from build123d import *

# Parameters (mm, degrees)
SKETCH1_W           = 14.7
SKETCH1_H           = 29.42
SKETCH1_R           = 1.5
SKETCH1_W_2         = 23
SKETCH1_H_2         = 35.5
BOSS_EXTRUDE5_DEPTH = 1.8
SKETCH2_W           = 23
SKETCH2_H           = 35.5
BOSS_EXTRUDE7_DEPTH = 2.6
SKETCH3_R           = 0.510447256
SKETCH3_R_2         = 0.580916902
SKETCH3_R_3         = 0.525090018
CUT_EXTRUDE1_DEPTH  = 1
SKETCH5_R           = 0.520017215
CUT_EXTRUDE5_DEPTH  = 1


with BuildPart() as part:
    # Sketch1 → Boss-Extrude5 (new body)
    # profile 1 of 3: a face of its own
    with BuildSketch(Plane.XY):
        Rectangle(SKETCH1_W, SKETCH1_H)
    # profile 2 of 3: a face of its own
    with BuildSketch(Plane.XY):
        Polygon((16.85, 17.75), (-16.85, 17.75), (-16.85, 3.519072364), (-12.987679058, 3.519072364), (-12.987679058, -4.65716191), (-16.85, -4.65716191), (-16.85, -17.75), (16.85, -17.75), align=None)
        with Locations((14.85, -15.71)):
            Circle(SKETCH1_R, mode=Mode.SUBTRACT)
        with Locations((14.85, 15.71)):
            Circle(SKETCH1_R, mode=Mode.SUBTRACT)
        with Locations((-14.85, 15.71)):
            Circle(SKETCH1_R, mode=Mode.SUBTRACT)
        with Locations((-14.85, -15.71)):
            Circle(SKETCH1_R, mode=Mode.SUBTRACT)
    # profile 3 of 3: a face of its own
    with BuildSketch(Plane.XY):
        Rectangle(SKETCH1_W_2, SKETCH1_H_2)
    extrude(amount=BOSS_EXTRUDE5_DEPTH)

    # Sketch2 → Boss-Extrude7 (add)
    with BuildSketch(Plane(origin=(0, 0, 0), x_dir=(-1, 0, 0), z_dir=(0, 0, -1))):
        Rectangle(SKETCH2_W, SKETCH2_H)
    extrude(amount=BOSS_EXTRUDE7_DEPTH)

    # Sketch3 → Cut-Extrude1 (cut)
    with BuildSketch(Plane(origin=(0, 0, 0), x_dir=(-1, 0, 0), z_dir=(0, 0, -1))):
        with Locations((-14.722097133, -5.610781363)):
            Circle(SKETCH3_R)
        with Locations((-14.722097133, -1.550914358)):
            Circle(SKETCH3_R_2)
        with Locations((-14.741724546, 2.500014567)):
            Circle(SKETCH3_R_3)
    extrude(amount=-CUT_EXTRUDE1_DEPTH, mode=Mode.SUBTRACT)

    # Sketch5 → Cut-Extrude5 (cut)
    with BuildSketch(Plane(origin=(0, 0, 0), x_dir=(-1, 0, 0), z_dir=(0, 0, -1))):
        with Locations((-14.677272087, 5.717301692)):
            Circle(SKETCH5_R)
    extrude(amount=-CUT_EXTRUDE5_DEPTH, mode=Mode.SUBTRACT)


solid = part.part
Verification items for the finished model (mm, model axes). A direction names the side the tool comes from. Round coordinates to 2 decimals unless told otherwise and drop trailing zeros. Loops run counter-clockwise (first coordinate to the right, second up) from the corner with the lowest first, then second, coordinate; pieces in that order, holes last. Notation, with made-up numbers: (38.5, 22) - (51.5, 22) arc R23 cw to (51.5, 42) - close; hole circle Ø11 at (42.25, 2.5). An arc over 180 degrees is marked (long way). Answer in a Markdown table with one row per item. Add a question column.
Q1. Gauge pin test, flat ends, axial feed: pin 1 (1 mm diameter, centred on y = -3.5, z = -1.5, fed in from -X); pin 2 (2 mm diameter, centred on y = -1.5, z = 0.5, fed in from -X); pin 3 (2.5 mm diameter, centred on x = 15.5, y = 4, fed in from -Z); pin 4 (2.5 mm diameter, centred on x = -14.85, y = 15.71, fed in from -Z). Record the tip position at first contact, or that the pin passes through.
Q2. Section check C-C on y = 4. Enter the section's corners in (x, z), plus the area to 3 significant figures.
Q3. Section check A-A on y = -15.71. Enter the section's corners in (x, z).
Q4. Section check D-D on z = -1.85. Enter the section's corners in (x, y), plus the area to 4 significant figures.
Q5. Section check B-B on x = -14.85. Enter the section's corners in (y, z), plus the area to 3 significant figures.
Q6. Material ranges on line 1 (Y direction, x = -14.85, z = 1.3); line 2 (X direction, y = 14.5, z = 0.8); line 3 (X direction, y = -12.5, z = -1.65), recorded low to high.
Q7. Release check for a two-part mould opening along Y. For faces 1 (the face through (-12.988, -1, 1)), 2 (the face through (-11.5, 0, -1)), 3 (the face through (0, -17.75, 0)) record: pulls with the +Y half, pulls with the -Y half, needs draft (parallel to the pull), parting line crosses it, or undercut.
Q8. Tool access check on faces 4 (the face through (-15, 3.519, 1)), 5 (the face through (14.7, -1.5, 1)), 6 (the face through (14, 0, 0)). Record the directions out of +Z, -Z, +X, -X, +Y, -Y that give a thin tool (end or side, any length) a straight path to the whole face; none if there is none.
Found:
| question | item | result |
|---|---|---|
| 1 | pin 1 | stops at x = -11.5 |
| 1 | pin 2 | stops at x = -12.99 |
| 1 | pin 3 | stops at z = 0 |
| 1 | pin 4 | passes through |
| 2 | outline | (-16.85, 0) - (-11.5, 0) - (-11.5, -2.6) - (11.5, -2.6) - (11.5, 0) - (16.85, 0) - (16.85, 1.8) - (-16.85, 1.8) - close |
| 2 | area | 120 mm² |
| 3 | outline | (-16.85, 0) - (-16.35, 0) - (-16.35, 1.8) - (-16.85, 1.8) - close; (-13.35, 0) - (-11.5, 0) - (-11.5, -2.6) - (11.5, -2.6) - (11.5, 0) - (13.35, 0) - (13.35, 1.8) - (-13.35, 1.8) - close; (16.35, 0) - (16.85, 0) - (16.85, 1.8) - (16.35, 1.8) - close |
| 4 | outline | (-11.5, -17.75) - (11.5, -17.75) - (11.5, 17.75) - (-11.5, 17.75) - close |
| 4 | area | 816.5 mm² |
| 5 | outline | (-17.75, 0) - (-17.21, 0) - (-17.21, 1.8) - (-17.75, 1.8) - close; (-14.21, 0) - (-4.66, 0) - (-4.66, 1.8) - (-14.21, 1.8) - close; (3.52, 0) - (14.21, 0) - (14.21, 1.8) - (3.52, 1.8) - close; (17.21, 0) - (17.75, 0) - (17.75, 1.8) - (17.21, 1.8) - close |
| 5 | area | 38.4 mm² |
| 6 | line 1 | y = -17.75 to -17.21, -14.21 to -4.66, 3.52 to 14.21, 17.21 to 17.75 |
| 6 | line 2 | x = -16.85 to -15.74, -13.96 to 13.96, 15.74 to 16.85 |
| 6 | line 3 | x = -11.5 to 11.5 |
| 7 | face 1 | undercut |
| 7 | face 2 | needs draft |
| 7 | face 3 | pulls with the -Y half |
| 8 | face 4 | +Z, -Z, -X |
| 8 | face 5 | -Z |
| 8 | face 6 | -Z, +X, +Y, -Y |
